```python
from build123d import *

# Parameters (mm, degrees)
SKETCH009_AS_DRAWN_R                      = 1.5
SKETCH009_AS_DRAWN_W                      = 51
SKETCH009_AS_DRAWN_H                      = 5.41
EXTRUDE010_DEPTH                          = 5
EXTRUDE010_ONTO_SKETCH009_PLACEMENT_ANGLE = 25.682094
SKETCH008_AS_DRAWN_R                      = 7
EXTRUDE009_DEPTH                          = 30
EXTRUDE009_ONTO_SKETCH008_PLACEMENT_ANGLE = 25.682094
SKETCH007_AS_DRAWN_R                      = 1.6
EXTRUDE008_DEPTH                          = 5
EXTRUDE008_ONTO_SKETCH007_PLACEMENT_ANGLE = 25.682094
EXTRUDE007_DEPTH                          = 100


with BuildPart() as extrude010:
    # Sketch009 as drawn → Extrude010 (new, symmetric)
    with BuildSketch(Plane.XY):
        with Locations((52, -10.02)):
            Circle(SKETCH009_AS_DRAWN_R)
        with Locations((77.5, -10.02)):
            Circle(SKETCH009_AS_DRAWN_R)
        with Locations((65.5, -5.585)):
            Rectangle(SKETCH009_AS_DRAWN_W, SKETCH009_AS_DRAWN_H)
    extrude(amount=EXTRUDE010_DEPTH, both=True)


with BuildPart() as extrude010_1:
    # Extrude010 onto Sketch009 placement: moved
    add(extrude010.part.moved(Location((0, -15.714438, 32.678321))).rotate(Axis((0, -15.714438, 32.678321), (1, 0, 0)), EXTRUDE010_ONTO_SKETCH009_PLACEMENT_ANGLE))


with BuildPart() as extrude009:
    # Sketch008 as drawn → Extrude009 (new)
    with BuildSketch(Plane.XY):
        with Locations((23.559155, -8.28634)):
            Circle(SKETCH008_AS_DRAWN_R)
    extrude(amount=-EXTRUDE009_DEPTH)


with BuildPart() as extrude009_1:
    # Extrude009 onto Sketch008 placement: moved
    add(extrude009.part.moved(Location((0, -15.714438, 32.678321))).rotate(Axis((0, -15.714438, 32.678321), (1, 0, 0)), EXTRUDE009_ONTO_SKETCH008_PLACEMENT_ANGLE))


with BuildPart() as extrude008:
    # Sketch007 as drawn → Extrude008 (new, symmetric)
    with BuildSketch(Plane.XY):
        with Locations((92.35981, 15.963995)):
            Circle(SKETCH007_AS_DRAWN_R)
        with Locations((7.880468, 15.845796)):
            Circle(SKETCH007_AS_DRAWN_R)
        with Locations((6.488905, -53.57334)):
            Circle(SKETCH007_AS_DRAWN_R)
        with Locations((93.218208, -53.681344)):
            Circle(SKETCH007_AS_DRAWN_R)
    extrude(amount=EXTRUDE008_DEPTH, both=True)


with BuildPart() as extrude008_1:
    # Extrude008 onto Sketch007 placement: moved
    add(extrude008.part.moved(Location((0, -15.714438, 32.678321))).rotate(Axis((0, -15.714438, 32.678321), (1, 0, 0)), EXTRUDE008_ONTO_SKETCH007_PLACEMENT_ANGLE))


with BuildPart() as tapa:
    # Sketch006 → Extrude007 (new body)
    with BuildSketch(Plane.YZ):
        Polygon((-65.452812, 5.76), (2.547146, 38.46), (2.547146, 41.46), (-65.452812, 8.76), align=None)
    extrude(amount=EXTRUDE007_DEPTH)

    # Cut004: cut Extrude008
    add(extrude008_1.part, mode=Mode.SUBTRACT)

    # Cut005: cut Extrude009
    add(extrude009_1.part, mode=Mode.SUBTRACT)

    # Cut006: cut Extrude010
    add(extrude010_1.part, mode=Mode.SUBTRACT)


solid = tapa.part
```
Input: part model. Units: mm. Frame: model coordinates. Give positions to 0.01 mm unless a question says otherwise; leave off trailing zeros. Order: outer loops, then holes, each group sorted by start corner. A loop starts at its lowest first (then second) coordinate and runs counter-clockwise, first axis right, second up. Notation, with made-up numbers: (-26, 13) - (4, 13) arc R19 cw to (4, 46) - close; hole circle Ø8 at (82.5, -1.75). An arc over 180 degrees is marked (long way). Use a Markdown table: item, result.
(1) Pin query (flat end, axial travel): pin 1 (8 mm diameter, centred on x = 64, z = 31, fed in from -Y); pin 2 (12 mm diameter, centred on x = 69.5, y = -44.5, fed in from -Z); pin 3 (2 mm diameter, centred on x = 49, y = -15, fed in from +Z); pin 4 (1.5 mm diameter, centred on y = -19, z = 33, fed in from -X). Return the tip coordinate at first contact, or that it passes through.
Computed values:
| item | result |
|---|---|
| pin 1 | stops at y = -27.52 |
| pin 2 | stops at z = 12.95 |
| pin 3 | stops at z = 33.5 |
| pin 4 | passes through |
(2) Line query: line 1 (Z direction, x = 21, y = -36.5); line 2 (Z direction, x = 16, y = -21.5); line 3 (Y direction, x = 29.5, z = 9). Output: solid intervals per line, ascending. Write a range as from..to.
Computed values:
| item | result |
|---|---|
| line 1 | z = 19.68..22.68 |
| line 2 | z = 26.9..29.9 |
| line 3 | y = -64.95..-58.72 |
(3) Section query D-D (z = 18). Output: boundary loops of the cut face in (x, y).
Computed values:
| item | result |
|---|---|
| outline | (0, -46.24) - (100, -46.24) - (100, -40) - (0, -40) - close |
(4) Section query A-A (x = 70.5). Output: boundary loops of the cut face in (y, z).
Computed values:
| item | result |
|---|---|
| outline | (-65.45, 5.76) - (-22.01, 26.65) - (-23.19, 29.09) - (-65.45, 8.76) - close; (-18.31, 31.43) - (-17.14, 28.99) - (2.55, 38.46) - (2.55, 41.46) - close |
(5) Section query C-C (y = -20). State how many separate pieces and enclosed holes the cut face has, then the cut area to 3 significant figures.
Computed values:
| item | result |
|---|---|
| separate pieces | 3 |
| enclosed holes | 0 |
| area | 109 mm2 |
(6) Draft query along Y for faces 1 (the cylindrical face through (94.744, -63.082, 8.421)), 2 (the flat face through (100, -32, 24)), 3 (the flat face through (49.3, -30.977, 25.339)). Return one class per face: released by +Y, released by -Y, zero draft, split by the parting line, or undercut.
Computed values:
| item | result |
|---|---|
| face 1 | undercut |
| face 2 | zero draft |
| face 3 | released by -Y |
(7) Section query B-B (x = 34). Output: boundary loops of the cut face in (y, z), then the cut area to 3 significant figures.
Computed values:
| item | result |
|---|---|
| outline | (-65.45, 5.76) - (2.55, 38.46) - (2.55, 41.46) - (-65.45, 8.76) - close |
| area | 204 mm2 |
